Geometry: final body of the model. Coordinates: model frame, mm. A direction names the side the tool comes from. Coordinates: 2 decimals unless noted, no trailing zeros.
from build123d import *

# Parameters (mm, degrees)
SKETCH_281X300_25_R   = 1.6
SKETCH_281X300_25_R_2 = 15
SKETCH_281X300_25_R_3 = 2.15
SKETCH_281X300_25_R_4 = 2.2
F_4MM_DEPTH           = 4


with BuildPart() as part:
    # 底板轮廓_281x300_安装孔外移25 → 凸台拉伸_4mm (new body)
    with BuildSketch(Plane.XY):
        with BuildLine():
            Line((-55.5, 108), (-55.5, 142))
            ThreePointArc((-55.5, 142), (-53.156854249, 147.656854249), (-47.5, 150))
            Line((-47.5, 150), (61.5, 150))
            ThreePointArc((61.5, 150), (67.156854249, 147.656854249), (69.5, 142))
            Line((69.5, 142), (69.5, 108))
            ThreePointArc((69.5, 108), (71.843145751, 102.343145751), (77.5, 100))
            Line((77.5, 100), (135.5, 100))
            ThreePointArc((135.5, 100), (139.035533906, 98.535533906), (140.5, 95))
            Line((140.5, 95), (140.5, -95))
            ThreePointArc((140.5, -95), (139.035533906, -98.535533906), (135.5, -100))
            Line((135.5, -100), (77.5, -100))
            ThreePointArc((77.5, -100), (71.843145751, -102.343145751), (69.5, -108))
            Line((69.5, -108), (69.5, -142))
            ThreePointArc((69.5, -142), (67.156854249, -147.656854249), (61.5, -150))
            Line((61.5, -150), (-47.5, -150))
            ThreePointArc((-47.5, -150), (-53.156854249, -147.656854249), (-55.5, -142))
            Line((-55.5, -142), (-55.5, -108))
            ThreePointArc((-55.5, -108), (-57.843145751, -102.343145751), (-63.5, -100))
            Line((-63.5, -100), (-127.5, -100))
            ThreePointArc((-127.5, -100), (-129.621320344, -99.121320344), (-130.5, -97))
            Line((-130.5, -97), (-130.5, -13))
            Line((-130.5, -13), (-130.5, 97))
            ThreePointArc((-130.5, 97), (-129.621320344, 99.121320344), (-127.5, 100))
            Line((-127.5, 100), (-63.5, 100))
            ThreePointArc((-63.5, 100), (-57.843145751, 102.343145751), (-55.5, 108))
        make_face()
        with Locations((100.5, -61)):
            Circle(SKETCH_281X300_25_R, mode=Mode.SUBTRACT)
        with Locations((130.5, -61)):
            Circle(SKETCH_281X300_25_R, mode=Mode.SUBTRACT)
        with Locations((100.5, 61)):
            Circle(SKETCH_281X300_25_R, mode=Mode.SUBTRACT)
        with Locations((7, 90.5)):
            Circle(SKETCH_281X300_25_R_2, mode=Mode.SUBTRACT)
        with Locations((7, 140)):
            Circle(SKETCH_281X300_25_R_3, mode=Mode.SUBTRACT)
        with Locations((-42.5, 90.5)):
            Circle(SKETCH_281X300_25_R_3, mode=Mode.SUBTRACT)
        with Locations((56.5, 90.5)):
            Circle(SKETCH_281X300_25_R_3, mode=Mode.SUBTRACT)
        with Locations((-40, 140)):
            Circle(SKETCH_281X300_25_R_3, mode=Mode.SUBTRACT)
        with Locations((130.5, 61)):
            Circle(SKETCH_281X300_25_R, mode=Mode.SUBTRACT)
        with Locations((7, 41)):
            Circle(SKETCH_281X300_25_R_3, mode=Mode.SUBTRACT)
        with Locations((31.290367902, -137.395183951)):
            Circle(SKETCH_281X300_25_R_4, mode=Mode.SUBTRACT)
        with Locations((-17.5, -137.395183951)):
            Circle(SKETCH_281X300_25_R_4, mode=Mode.SUBTRACT)
        with Locations((-17.5, -88.604816049)):
            Circle(SKETCH_281X300_25_R_4, mode=Mode.SUBTRACT)
        with Locations((31.290367902, -88.604816049)):
            Circle(SKETCH_281X300_25_R_4, mode=Mode.SUBTRACT)
        with Locations((7, 111.5)):
            Circle(SKETCH_281X300_25_R, mode=Mode.SUBTRACT)
        with Locations((25.186533479, 101)):
            Circle(SKETCH_281X300_25_R, mode=Mode.SUBTRACT)
        with Locations((100.5, -91)):
            Circle(SKETCH_281X300_25_R, mode=Mode.SUBTRACT)
        with Locations((25.186533479, 80)):
            Circle(SKETCH_281X300_25_R, mode=Mode.SUBTRACT)
        with Locations((100.5, 91)):
            Circle(SKETCH_281X300_25_R, mode=Mode.SUBTRACT)
        with Locations((7, 69.5)):
            Circle(SKETCH_281X300_25_R, mode=Mode.SUBTRACT)
        with Locations((130.5, 91)):
            Circle(SKETCH_281X300_25_R, mode=Mode.SUBTRACT)
        with Locations((130.5, -91)):
            Circle(SKETCH_281X300_25_R, mode=Mode.SUBTRACT)
        with Locations((-43, -105)):
            Circle(SKETCH_281X300_25_R, mode=Mode.SUBTRACT)
        with Locations((57, -57)):
            Circle(SKETCH_281X300_25_R, mode=Mode.SUBTRACT)
        with Locations((-43, -57)):
            Circle(SKETCH_281X300_25_R, mode=Mode.SUBTRACT)
        with Locations((57, -105)):
            Circle(SKETCH_281X300_25_R, mode=Mode.SUBTRACT)
        with Locations((-11.186533479, 80)):
            Circle(SKETCH_281X300_25_R, mode=Mode.SUBTRACT)
        with Locations((-11.186533479, 101)):
            Circle(SKETCH_281X300_25_R, mode=Mode.SUBTRACT)
        with Locations((130.5, 10)):
            Circle(SKETCH_281X300_25_R, mode=Mode.SUBTRACT)
        with Locations((130.5, -10)):
            Circle(SKETCH_281X300_25_R, mode=Mode.SUBTRACT)
        with Locations((-120.5, 10)):
            Circle(SKETCH_281X300_25_R, mode=Mode.SUBTRACT)
        with Locations((-120.5, -10)):
            Circle(SKETCH_281X300_25_R, mode=Mode.SUBTRACT)
        with Locations((-43, -115)):
            Circle(SKETCH_281X300_25_R, mode=Mode.SUBTRACT)
        with Locations((57, -67)):
            Circle(SKETCH_281X300_25_R, mode=Mode.SUBTRACT)
        with Locations((57, -115)):
            Circle(SKETCH_281X300_25_R, mode=Mode.SUBTRACT)
        with Locations((-43, -67)):
            Circle(SKETCH_281X300_25_R, mode=Mode.SUBTRACT)
        with Locations((-120.5, -91)):
            Circle(SKETCH_281X300_25_R, mode=Mode.SUBTRACT)
        with Locations((-90.5, -91)):
            Circle(SKETCH_281X300_25_R, mode=Mode.SUBTRACT)
        with Locations((-120.5, 91)):
            Circle(SKETCH_281X300_25_R, mode=Mode.SUBTRACT)
        with Locations((-90.5, 91)):
            Circle(SKETCH_281X300_25_R, mode=Mode.SUBTRACT)
        with Locations((-90.5, 61)):
            Circle(SKETCH_281X300_25_R, mode=Mode.SUBTRACT)
        with Locations((-120.5, 61)):
            Circle(SKETCH_281X300_25_R, mode=Mode.SUBTRACT)
        with Locations((-90.5, -61)):
            Circle(SKETCH_281X300_25_R, mode=Mode.SUBTRACT)
        with Locations((-120.5, -61)):
            Circle(SKETCH_281X300_25_R, mode=Mode.SUBTRACT)
        with Locations((130.5, 43)):
            Circle(SKETCH_281X300_25_R, mode=Mode.SUBTRACT)
        with Locations((130.5, -43)):
            Circle(SKETCH_281X300_25_R, mode=Mode.SUBTRACT)
        with Locations((-120.5, 43)):
            Circle(SKETCH_281X300_25_R, mode=Mode.SUBTRACT)
        with Locations((-120.5, -43)):
            Circle(SKETCH_281X300_25_R, mode=Mode.SUBTRACT)
        with Locations((52, 140)):
            Circle(SKETCH_281X300_25_R_3, mode=Mode.SUBTRACT)
        with Locations((-40, -140)):
            Circle(SKETCH_281X300_25_R_3, mode=Mode.SUBTRACT)
        with Locations((52, -140)):
            Circle(SKETCH_281X300_25_R_3, mode=Mode.SUBTRACT)
        with BuildLine():
            Line((-25.5, -97), (-25.5, -129))
            ThreePointArc((-25.5, -129), (-24.914213562, -130.414213562), (-23.5, -131))
            Line((-23.5, -131), (42.5, -131))
            ThreePointArc((42.5, -131), (43.914213562, -130.414213562), (44.5, -129))
            Line((44.5, -129), (44.5, -97))
            ThreePointArc((44.5, -97), (43.914213562, -95.585786438), (42.5, -95))
            Line((42.5, -95), (-23.5, -95))
            ThreePointArc((-23.5, -95), (-24.914213562, -95.585786438), (-25.5, -97))
        make_face(mode=Mode.SUBTRACT)
        with BuildLine():
            Line((75.5, 50), (75.5, 36))
            ThreePointArc((75.5, 36), (80.5, 31), (85.5, 36))
            Line((85.5, 36), (85.5, 50))
            ThreePointArc((85.5, 50), (80.5, 55), (75.5, 50))
        make_face(mode=Mode.SUBTRACT)
        with BuildLine():
            Line((85.5, -50), (85.5, -36))
            ThreePointArc((85.5, -36), (80.5, -31), (75.5, -36))
            Line((75.5, -36), (75.5, -50))
            ThreePointArc((75.5, -50), (80.5, -55), (85.5, -50))
        make_face(mode=Mode.SUBTRACT)
        with BuildLine():
            Line((-95.5, -10), (-75.5, -10))
            ThreePointArc((-75.5, -10), (-65.5, 0), (-75.5, 10))
            Line((-75.5, 10), (-95.5, 10))
            ThreePointArc((-95.5, 10), (-105.5, 0), (-95.5, -10))
        make_face(mode=Mode.SUBTRACT)
    extrude(amount=F_4MM_DEPTH)


solid = part.part
Item 1: Section A-A, the plane z = 1.9. State how many separate pieces and enclosed holes the cut face has, plus the area to 3 significant figures.
Derived:
separate pieces: 1
enclosed holes: 55
area: 61,800 mm2
Item 2: Material intervals for probe 1 along Y at (x, z) = (25.5, 0.4); probe 2 along X at (y, z) = (-67, 1.1); probe 3 along X at (y, z) = (140, 2.9), sorted ascending.
Derived:
probe 1: y = -150 to -131, -95 to 78.43, 81.57 to 99.43, 102.57 to 150
probe 2: x = -130.5 to -44.6, -41.4 to 55.4, 58.6 to 140.5
probe 3: x = -55.5 to -42.15, -37.85 to 4.85, 9.15 to 49.85, 54.15 to 69.5
Item 3: Set-up query: faces 1 (the cylindrical face through (-53.219, 147.594, 1.972)), 2 (the cylindrical face through (-65.5, -0.2, 2)). Return all of +Z, -Z, +X, -X, +Y, -Y with unobstructed straight access to the full face (end or side cutting, diameter ignored); none if empty.
Derived:
face 1: +Z, -Z, -X, +Y
face 2: +Z, -Z
Item 4: Pin query (flat end, axial travel): pin 1 (1.5 mm diameter, centred on x = 100.5, z = 2.5, fed in from +Y); pin 2 (2.5 mm diameter, centred on x = 52, y = -140, fed in from +Z); pin 3 (1.2 mm diameter, centred on x = -84.5, z = 1, fed in from -Y); pin 4 (1.2 mm diameter, centred on y = -118.5, z = 2.5, fed in from -X). Return the tip coordinate at first contact, or that it passes through.
Derived:
pin 1: stops at y = 100
pin 2: passes through
pin 3: stops at y = -100
pin 4: stops at x = -55.5
Item 5: Pull-direction query (Y, two-part tool) for faces 3 (the flat face through (7, 2, 4)), 4 (the cylindrical face through (3.748, 75.857, 1.972)), 5 (the cylindrical face through (71.781, 102.406, 1.972)); classes: released by +Y, released by -Y, zero draft, split by the parting line, or undercut.
Derived:
face 3: zero draft
face 4: undercut
face 5: released by +Y
